Autodesk Fusion 360 part; units mm, degrees
sketch "main body" plane through (0, 0, 0) normal (0, 1, 0) x (1, 0, 0) in component "main"
  arc A0 (-7.5849, 2.5435) -> (7.6843, 2.225) centre (0, 0) ccw
  line L0 (-7.5849, 2.5435) -> (-38.6454, -15.3377)
  line L1 (-38.6454, -15.3377) -> (-0.1069, 25.2491)
  line L2 (-0.1069, 25.2491) -> (39.4777, -14.3181)
  line L3 (39.4777, -14.3181) -> (7.6843, 2.225)
  dimension "d1" = 8
extrude "Extrude1" add sketch "main body" along normal blind 20 in component "main"
fillet "Fillet1" radius 15 1 edges at (-0.1069, 10, -25.2491) in component "main"
sketch "main hole" plane through (0, 20, 0) normal (0, 1, 0) x (-1, 0, 0) in component "main"
  arc A0 (-10.7778, -14.3691) -> (10.704, -14.0888) centre (-0.1736, -3.7602) ccw
  line L0 (10.704, -14.0888) -> (38.6454, 15.3377)
  line L1 (38.6454, 15.3377) -> (7.5849, -2.5435)
  line L2 (-7.6843, -2.225) -> (-39.4777, 14.3181)
  line L3 (-39.4777, 14.3181) -> (-10.7778, -14.3691)
  circle A1 centre (-0.0035, 1.6197) radius 6.5
  line L4 (-10.0035, 3.8921) -> (9.9387, 3.8921)
  line L5 (9.9387, 3.8921) -> (9.9387, 20.1413)
  line L6 (9.9387, 20.1413) -> (-10.0035, 20.1413)
  line L7 (-10.0035, 20.1413) -> (-10.0035, 3.8921)
  line L8 (-10.0035, 3.8921) -> (9.9387, 20.1413) construction
  line L9 (9.9387, 3.8921) -> (-10.0035, 20.1413) construction
  dimension "d5" = 13
extrude "Extrude5" cut sketch "main hole" against normal blind 20 in component "main"
extrude "Extrude3" cut sketch "main hole" against normal blind 20 contours A1 L4 | A1 L4 in component "main"
sketch "rounded borders" plane through (0, 0, 0) normal (0, 1, 0) x (1, 0, 0) in component "main"
  circle A0 centre (-7.8046, -4.9719) radius 2
  circle A1 centre (7.7907, -4.9961) radius 2
  dimension "d16" = 4
  dimension "d17" = 4
extrude "Extrude6" add sketch "rounded borders" along normal blind 20 in component "main"
sketch "cut sides" plane through (0, 0, 0) normal (1, 0, 0) x (0, 0, -1) in component "main"
  line L0 (28, 22) -> (-17, 12)
  line L1 (-15.3377, 0) -> (-15.3377, 20)
  line L2 (-17, 12) -> (-17, 22)
  line L3 (-17, 22) -> (28, 22)
  line L4 (28, -2) -> (-17, 8)
  line L5 (-17, 8) -> (-17, -2)
  line L6 (-17, -2) -> (28, -2)
extrude "Extrude7" cut sketch "cut sides" along normal mid plane 100 in component "main"
sketch "Sketch9" plane through (0, 0, 0) normal (1, 0, 0) x (0, 1, 0) in component "main"
  circle A0 centre (10, -18.5) radius 0.825
  dimension "d22" = 1.65
extrude "Extrude8" cut sketch "Sketch9" along normal mid plane 40 in component "main"
component "main" placed x (1, 0, 0) y (0, 1, 0) z (0, 0, 1) at (0, 0, 0)
properties part number "rampClip"
Source: CAD feature listing. Evaluate the final solid. Frame: model axes, mm. A direction names the side the tool comes from. Round coordinates to 2 decimals unless told otherwise and drop trailing zeros. Loops run counter-clockwise (first coordinate to the right, second up) from the corner with the lowest first, then second, coordinate; pieces in that order, holes last. Notation, with made-up numbers: (10.25, 79.5) - (50.25, 79.5) arc R33 ccw to (50.25, 112.5) - close; hole circle Ø1 at (3, -22). An arc over 180 degrees is marked (long way). Use CSV: the item, a comma, the result in double quotes.
Q1. Pin query (flat end, axial travel): pin 1 Ø4 at (y, z) = (16, -12.5) entering from +X; pin 2 Ø10 at (y, z) = (9.5, 1.5) entering from +X; pin 3 Ø1.3 at (y, z) = (10, -18.5) entering from +X; pin 4 Ø6 at (x, z) = (4.5, -12.5) entering from +Y. Return the tip coordinate at first contact, or that it passes through.
Reported:
pin 1,"x = 14.65"
pin 2,"x = 31.66"
pin 3,"through"
pin 4,"y = 19.22"
Q2. Section query D-D, the plane x = -25. Output: boundary loops of the cut face in (y, z), then the cut area to 3 significant figures.
Reported:
outline,"(4.44, 0.97) - (15.56, 0.97) - (14.12, 7.48) - (5.88, 7.48) - close"
area,"63.1 mm^2"
Q3. Mould query, pull axis Z, two halves, no side actions, for faces 1 (the cylindrical face through (9.68, 9.93, 5.65)), 2 (the flat face through (3.127, 2.982, -5.579)), 3 (the cylindrical face through (8, 10, 0)), 4 (the flat face through (-21.766, 9.875, -2.439)). Classes: pulls with the +Z half, pulls with the -Z half, needs draft (parallel to the pull), parting line crosses it, or undercut.
Reported:
face 1,"undercut"
face 2,"pulls with the +Z half"
face 3,"undercut"
face 4,"pulls with the -Z half"
Q4. Reachability of faces 5 (the flat face through (-19.447, 9.911, 4.285)), 6 (the flat face through (21.74, 9.87, -3.41)) from +Z, -Z, +X, -X, +Y, -Y: full face, straight path, thin tool, end or side. Return the list, or none.
Reported:
face 5,"+Y, -Y"
face 6,"-Z, +X, +Y, -Y"
Q5. Section query A-A, the plane z = 5. Output: boundary loops of the cut face in (x, y), then the cut area to 3 significant figures.
Reported:
outline,"(-28.83, 5.33) - (-20.69, 5.33) - (-20.69, 14.67) - (-28.83, 14.67) - close; (-9.8, 5.33) - (-5.8, 5.33) - (-5.8, 14.67) - (-9.8, 14.67) - close; (5.79, 5.33) - (9.79, 5.33) - (9.79, 14.67) - (5.79, 14.67) - close; (21.57, 5.33) - (30.16, 5.33) - (30.16, 14.67) - (21.57, 14.67) - close"
area,"231 mm^2"
Q6. Section query C-C, the plane z = -4. Output: boundary loops of the cut face in (x, y).
Reported:
outline,"(-20.28, 3.33) - (-3.26, 3.33) - (-3.26, 16.67) - (-20.28, 16.67) - close; (3.27, 3.33) - (21.15, 3.33) - (21.15, 16.67) - (3.27, 16.67) - close"
Q7. Ray query, line 1 along X through (y, z) = (8, 5.5); line 2 along X through (y, z) = (14, 6.5); line 3 along X through (y, z) = (14.5, -3). Return the intervals inside material, ascending.
Reported:
line 1,"-29.3 to -21.56, -9.73 to -5.88, 5.86 to 9.73, 22.53 to 30.66"
line 2,"-30.25 to -23.29, -9.09 to -6.51, 6.47 to 9.11, 24.45 to 31.66"
line 3,"-21.23 to -4.57, 4.58 to 22.15"
